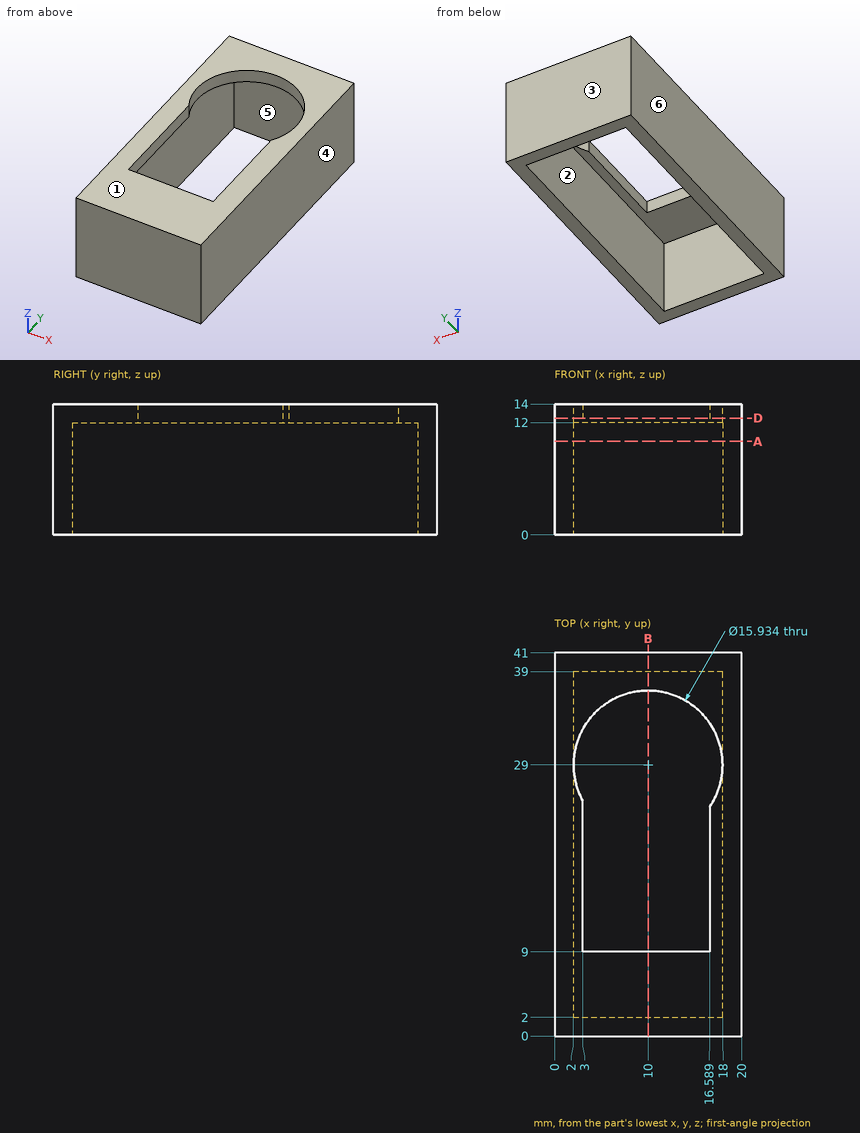
Print and shaded views of the part. All mm, measured from the part's lowest x, y and z. A direction names the side the tool comes from. Coordinates: 2 decimals unless noted, no trailing zeros. Loops run counter-clockwise (first coordinate to the right, second up) from the corner with the lowest first, then second, coordinate; pieces in that order, holes last. Notation, with made-up numbers: M -38,80 L -31,80 A28 ccw -31,118 Z; hole C 89,51.25 d10. An arc over 180 degrees is marked long. Use a Markdown table: item, result. Add a question column.
Q1. Cut at D-D (z = 12.5). Write the cut outline in (x, y) (1 decimal).
Q2. Mould opens along X. For the marked faces 3, 4, 5 and 6 say: +X half, -X half, draft (parallel to the pull), parting line (faces both ways), or undercut.
Q3. Cut at B-B (x = 10). Write the cut outline in (y, z).
Q4. Which spindle directions (+Z, -Z, +X, -X, +Y, -Y) get a long thin tool onto all of the face, cutting with end or side? Do the marked faces 1 and 2. Say none if no direction does.
Q5. Cut at A-A (z = 10). Write the cut outline in (x, y), and give its area (3 significant figures).
Q6. Pin check, flat tip, straight feed: P1, Ø5, axis at x = 15, y = 5.5, coming from the -Z side. Stop position of the tip, or through.
Q7. Probe L1, parallel to X at y = 31.5, z = 9.75; L2, parallel to X at y = 9.5, z = 13; L3, parallel to Y at x = 5, z = 10.75. List the from-to ranges inside material, lowest first.
Worked out:
| question | item | result |
|---|---|---|
| 1 | outline | M 0,0 L 20,0 L 20,41 L 0,41 Z; hole M 3,9 L 16.6,9 L 16.6,24.5 A8 ccw long 3,25.2 Z |
| 2 | face 3 | draft |
| 2 | face 4 | +X half |
| 2 | face 5 | undercut |
| 2 | face 6 | -X half |
| 3 | outline | M 0,0 L 2,0 L 2,12 L 9,12 L 9,14 L 0,14 Z; M 36.97,12 L 39,12 L 39,0 L 41,0 L 41,14 L 36.97,14 Z |
| 4 | face 1 | +Z, +X, -X, +Y, -Y |
| 4 | face 2 | -Z |
| 5 | outline | M 0,0 L 20,0 L 20,41 L 0,41 Z; hole M 2,2 L 18,2 L 18,39 L 2,39 Z |
| 5 | area | 228 mm2 |
| 6 | P1 | stops at z = 12 |
| 7 | L1 | x = 0 to 2, 18 to 20 |
| 7 | L2 | x = 0 to 3, 16.59 to 20 |
| 7 | L3 | y = 0 to 2, 39 to 41 |
